Work out the finished part from the listing and answer in its coordinate system (mm). Face numbers are marked on the shaded views. A direction names the side the tool comes from. Coordinates: 2 decimals unless noted, no trailing zeros. Order: outer loops, then holes, each group sorted by start corner. A loop starts at its lowest first (then second) coordinate and runs counter-clockwise, first axis right, second up. Notation, with made-up numbers: M 66.5,76.5 L 119.5,76.5 A20 cw 119.5,105.5 Z; hole C 43.5,55.5 d2. An arc over 180 degrees is marked long. Answer in a Markdown table with one row per item. Add a question column.
Item 1: The mould has two halves that part along Y. Classify the marked faces 3 and 4: released by +Y, released by -Y, zero draft, split by the parting line, or undercut.
Item 2: Which of the six approach directions +Z, -Z, +X, -X, +Y, -Y give full straight-line access (tool end or side, diameter ignored) to the marked faces 1 and 2?
Item 3: The part is cut by section B-B (x = 0). Write down the section's boundary in (y, z), then the cut area to 3 significant figures.
Item 4: Flat-ended cylindrical pins translate along their axes: pin 1 Ø0.5 at (y, z) = (-58.5, 38) entering from -X; pin 2 Ø3 at (x, z) = (-1, 34) entering from +Y; pin 3 Ø2 at (x, y) = (-2, -11.5) entering from +Z. Find the tip coordinate at first contact, or state that the pin passes through.
Item 5: The part is cut by section A-A (y = -47). Write down the section's boundary in (x, z), then the cut area to 3 significant figures.
Item 6: Consider line 1 (Y direction, x = -0.25, z = 34.5); line 2 (Y direction, x = -0.75, z = 32.25); line 3 (Z direction, x = -2.5, y = -38). Determine where each line is inside the solid, lowest interval first. Write a range as from..to.
from build123d import *

# Parameters (mm, degrees)
BOSS_EXTRUDE2_DEPTH = 75.5
BOSS_EXTRUDE3_DEPTH = 85.5
SKETCH7_W           = 37.5
SKETCH7_H           = 5
SKETCH9_R           = 1.55
CUT_EXTRUDE4_DEPTH  = 4.3
SKETCH10_R          = 2.4
CUT_EXTRUDE5_DEPTH  = 0.5
SKETCH13_R          = 2.4
CUT_EXTRUDE6_DEPTH  = 0.5
SKETCH14_R          = 1.55
CUT_EXTRUDE7_DEPTH  = 4.3


with BuildPart() as part:
    # Sketch3 → Boss-Extrude2 (new body)
    with BuildSketch(Plane.XZ.offset(5)):
        with BuildLine():
            Line((-3, 37.379807383), (-3, 31.379807383))
            Line((-3, 31.379807383), (3, 31.379807383))
            Line((3, 31.379807383), (3, 37.379807383))
            ThreePointArc((3, 37.379807383), (0, 37.5), (-3, 37.379807383))
        make_face()
    extrude(amount=BOSS_EXTRUDE2_DEPTH)

    # Sketch5 → Boss-Extrude3 (add)
    with BuildSketch(Plane(origin=(0, 0, 0), x_dir=(1, 0, 0), z_dir=(0, 1, 0))):
        with BuildLine():
            Line((-2.99999884, -38.360165319), (-2.99999884, -39.385911275))
            ThreePointArc((-2.99999884, -39.385911275), (1.163e-06, -39.5), (3.00000116, -39.385911098))
            Line((3.00000116, -39.385911098), (3.00000116, -38.381035126))
            ThreePointArc((3.00000116, -38.381035126), (2.500212929, -38.41682964), (2.00000116, -38.446116314))
            Line((2.00000116, -38.446116314), (2.00000116, -37.446628625))
            ThreePointArc((2.00000116, -37.446628625), (0, -37.5), (-2.00000116, -37.446628625))
            Line((-2.00000116, -37.446628625), (-2.00000116, -38.425281674))
            ThreePointArc((-2.00000116, -38.425281674), (-2.500211998, -38.395979168), (-2.99999884, -38.360165319))
        make_face()
    extrude(amount=-BOSS_EXTRUDE3_DEPTH)

    # Sketch7 → Cut-Revolve1 (revolve, cut)
    with BuildSketch(Plane(origin=(0, 0, 0), x_dir=(0, 0, -1), z_dir=(1, 0, 0))):
        with Locations((-18.75, -64)):
            Rectangle(SKETCH7_W, SKETCH7_H)
    revolve(axis=Axis((0, -27.016689378, 0), (0, -1, 0)), mode=Mode.SUBTRACT)

    # Sketch9 → Cut-Extrude4 (cut)
    with BuildSketch(Plane(origin=(0, -80.5, 0), x_dir=(-1, 0, 0), z_dir=(0, -1, 0))):
        with Locations((0, -34.420864201)):
            Circle(SKETCH9_R)
    extrude(amount=-CUT_EXTRUDE4_DEPTH, mode=Mode.SUBTRACT)

    # Sketch10 → Cut-Extrude5 (cut)
    with BuildSketch(Plane(origin=(0, -80.5, 0), x_dir=(-1, 0, 0), z_dir=(0, -1, 0))):
        with Locations((0, -34.420864201)):
            Circle(SKETCH10_R)
    extrude(amount=-CUT_EXTRUDE5_DEPTH, mode=Mode.SUBTRACT)

    # Sketch13 → Cut-Extrude6 (cut)
    with BuildSketch(Plane(origin=(0, -5, 0), x_dir=(-1, 0, 0), z_dir=(0, -1, 0))):
        with Locations((0, -34.379807383)):
            Circle(SKETCH13_R)
    extrude(amount=CUT_EXTRUDE6_DEPTH, mode=Mode.SUBTRACT)

    # Sketch14 → Cut-Extrude7 (cut)
    with BuildSketch(Plane(origin=(0, -5, 0), x_dir=(-1, 0, 0), z_dir=(0, -1, 0))):
        with Locations((0, -34.379807383)):
            Circle(SKETCH14_R)
    extrude(amount=CUT_EXTRUDE7_DEPTH, mode=Mode.SUBTRACT)


solid = part.part
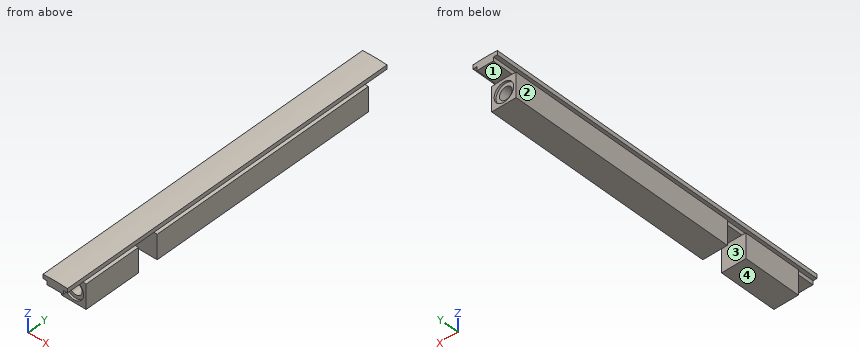
Reply:
| question | item | result |
|---|---|---|
| 1 | face 3 | undercut |
| 1 | face 4 | zero draft |
| 2 | face 1 | -Z, +Y |
| 2 | face 2 | +Z, -Z, -X, +Y, -Y |
| 3 | outline | M -85.5,37.5 L -80.5,37.5 L -80.5,36.82 L -80,36.82 L -80,35.97 L -76.2,35.97 L -76.2,32.87 L -80,32.87 L -80,32.02 L -80.5,32.02 L -80.5,31.38 L -66.5,31.38 L -66.5,37.5 L -61.5,37.5 L -61.5,31.38 L -5,31.38 L -5,31.98 L -5.5,31.98 L -5.5,32.83 L -9.3,32.83 L -9.3,35.93 L -5.5,35.93 L -5.5,36.78 L -5,36.78 L -5,37.5 L 0,37.5 L 0,39.5 L -85.5,39.5 Z |
| 3 | area | 574 mm2 |
| 4 | pin 1 | stops at x = -2 |
| 4 | pin 2 | stops at y = -5 |
| 4 | pin 3 | stops at z = 39.49 |
| 5 | outline | M -3,31.38 L 3,31.38 L 3,37.38 A37.5 ccw 2,37.45 L 2,38.45 A38.5 cw 3,38.38 L 3,39.39 A39.5 ccw -3,39.39 L -3,38.36 A38.48 cw -2,38.43 L -2,37.45 A37.5 ccw -3,37.38 Z |
| 5 | area | 46.5 mm2 |
| 6 | line 1 | y = -76.2..-66.5, -61.5..-9.3 |
| 6 | line 2 | y = -80..-66.5, -61.5..-5.5 |
| 6 | line 3 | z = 31.38..37.42, 38.4..39.42 |
